Here's the drawing with two shaded views (mm, measured from the low corner). I have some questions. Give positions to 0.01 mm unless a question says otherwise; leave off trailing zeros. Order: outer loops, then holes, each group sorted by start corner. A loop starts at its lowest first (then second) coordinate and runs counter-clockwise, first axis right, second up. Notation, with made-up numbers: M -8,74 L 0,74 A28 ccw 0,97 Z; hole C -36,27.5 d10. An arc over 180 degrees is marked long. Write each question's results on one line, items separated by ' | '.
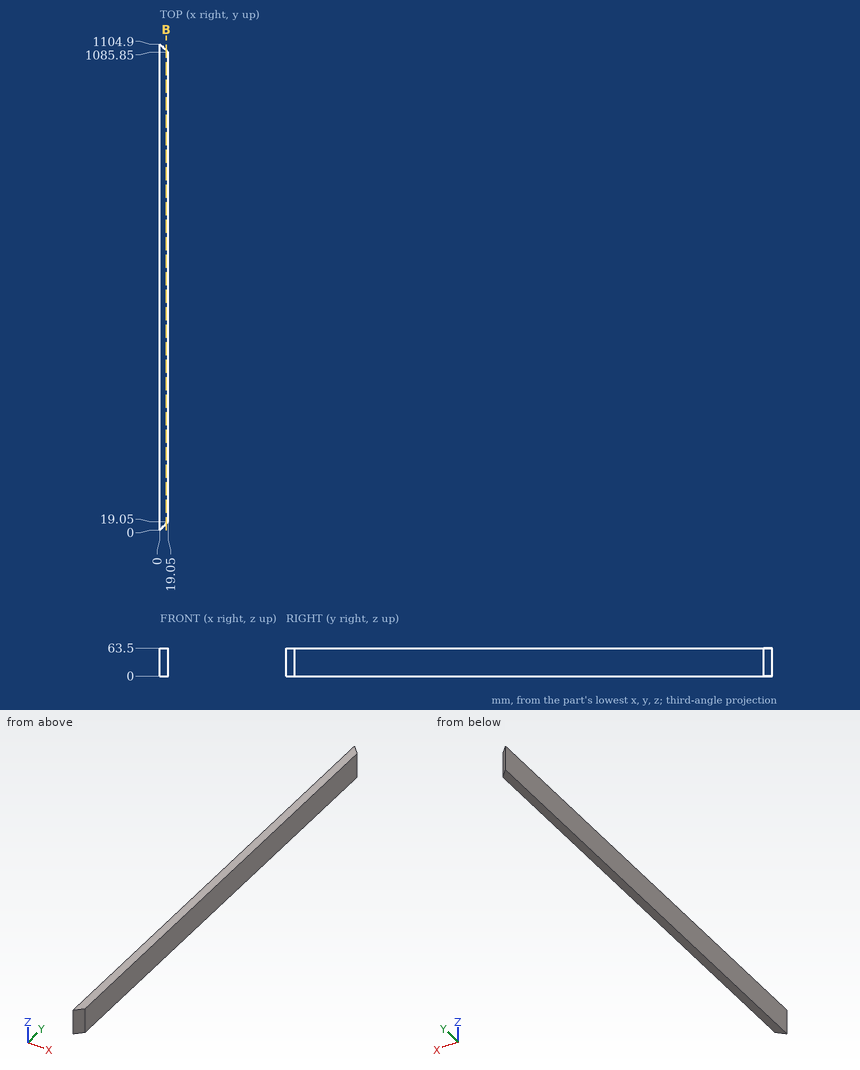
(1) Will these pins go through, and if not, where does the flat tip stop? P1, Ø10, axis at x = 15.5, z = 41, coming from the -Y side; P2, Ø4, axis at x = 3.5, y = 446.5, coming from the -Z side.
Data:
P1: stops at y = 10.5 | P2: stops at z = 0
(2) Imagine slicing it at B-B, the plane x = 14.5. Write out the boundary of the cut face in (y, z).
Data:
outline: M 14.5,0 L 1090.4,0 L 1090.4,63.5 L 14.5,63.5 Z
(3) I need wall thicknesses on L1, parallel to Y at x = 15.5, z = 57; L2, parallel to Y at x = 5.5, z = 30. Which ranges of each line are inside material? Lowest first, please. Write a range as from..to.
Data:
L1: y = 15.5..1089.4 | L2: y = 5.5..1099.4
